The model under review builds one solid part; all positions refer to its coordinate system, in mm. A direction names the side the tool comes from. Give positions to 0.01 mm unless a question says otherwise; leave off trailing zeros. Loops run counter-clockwise (first coordinate to the right, second up) from the corner with the lowest first, then second, coordinate; pieces in that order, holes last. Notation, with made-up numbers: (-9.5, -24.5) - (8.5, -24.5) arc R25 ccw to (8.5, -10.5) - close; hole circle Ø10 at (-6.5, 74.25). An arc over 180 degrees is marked (long way). Answer as a JSON object with one key per item and string values.
from build123d import *


# Not quite as in the source:
# - a feature names something its author has since deleted; it is built from what else it names


with BuildPart() as f2:
    # F2: sweep along a path in F0
    with BuildLine(Plane.XY) as f2_path:
        Line((-7.5, -8.5), (-7.5, 8.5))
        ThreePointArc((-7.5, 8.5), (-6.0355339059, 12.0355339059), (-2.5, 13.5))
        Line((-2.5, 13.5), (2.5, 13.5))
        ThreePointArc((2.5, 13.5), (6.0355339059, 12.0355339059), (7.5, 8.5))
        Line((7.5, 8.5), (7.5, -8.5))
        ThreePointArc((7.5, -8.5), (6.0355339059, -12.0355339059), (2.5, -13.5))
        Line((2.5, -13.5), (-2.5, -13.5))
        ThreePointArc((-2.5, -13.5), (-6.0355339059, -12.0355339059), (-7.5, -8.5))
    # F1 (on Front) → F2 (sweep)
    with BuildSketch(Plane.XZ):
        Polygon((-5.751425866, 1.454347861), (-6.6942584633, 1.8659339551), (-9.2492606491, 1.454347861), (-9.3934396282, 0), (-9.2492606491, -1.454347861), (-6.6942584633, -1.8659339551), (-5.751425866, -1.454347861), (-5.751425866, 0), align=None)
    sweep(path=f2_path.line)


solid = f2.part
Q1. Consider section D-D, the plane z = -0.8. State the section outline as (x, y) points, plus the area to 3 significant figures.
Results:
{"outline": "(-9.31, -8.5) arc R6.81 ccw to (-2.5, -15.31) - (2.5, -15.31) arc R6.81 ccw to (9.31, -8.5) - (9.31, 8.5) arc R6.81 ccw to (2.5, 15.31) - (-2.5, 15.31) arc R6.81 ccw to (-9.31, 8.5) - close; hole (-5.75, -8.5) arc R3.25 ccw to (-2.5, -11.75) - (2.5, -11.75) arc R3.25 ccw to (5.75, -8.5) - (5.75, 8.5) arc R3.25 ccw to (2.5, 11.75) - (-2.5, 11.75) arc R3.25 ccw to (-5.75, 8.5) - close", "area": "269 mm^2"}
Q2. Clearance check with flat-ended pins moving along their axes: pin 1 Ø2 at (x, y) = (5.5, -7) entering from +Z; pin 2 Ø8 at (x, y) = (-5, -3.5) entering from -Z; pin 3 Ø1 at (x, z) = (6.5, 1) entering from -Y. State where each tip first meets the part, or that it passes through.
Results:
{"pin 1": "stops at z = 1.78", "pin 2": "stops at z = -1.87", "pin 3": "stops at y = -14.33"}
Q3. Consider section A-A, the plane y = 5. State the section outline as (x, z) points, plus the area to 3 significant figures.
Results:
{"outline": "(-9.39, 0) - (-9.25, -1.45) - (-6.69, -1.87) - (-5.75, -1.45) - (-5.75, 1.45) - (-6.69, 1.87) - (-9.25, 1.45) - close; (5.75, -1.45) - (6.69, -1.87) - (9.25, -1.45) - (9.39, 0) - (9.25, 1.45) - (6.69, 1.87) - (5.75, 1.45) - close", "area": "23.6 mm^2"}
Q4. For faces 1 (the face through (-4.8, 10.8, 0)), 2 (the face through (-5.94, -12.02, 1.75)), 3 (the face through (-0.035, -12.229, -1.663)), list the 3-axis set-ups (+Z, -Z, +X, -X, +Y, -Y) from which the entire face can be reached by the end or side of a thin tool; tool diameter is ignored.
Results:
{"face 1": "+Z, -Z", "face 2": "+Z, -X, -Y", "face 3": "-Z"}
Q5. To check wall thickness, follow probe 1 along X at (y, z) = (6, -0.55); probe 2 along X at (y, z) = (-9, 1.2); probe 3 along Y at (x, z) = (5.25, -0.1). State the ranges of each line that lie inside material, in increasing order. Write a range as [from, to].
Results:
{"probe 1": "x = [-9.34, -5.75], [5.75, 9.34]", "probe 2": "x = [-9.26, -5.71], [5.71, 9.26]", "probe 3": "y = [-14.81, -10.23], [10.23, 14.81]"}
Q6. The part is to be moulded in two halves that separate along Y. For faces 4 (the face through (4.8, -10.8, 0)), 5 (the face through (-0.03, -15.32, 0.74)), 6 (the face through (5.917, 11.993, -1.754)), say which applies: +Y half, -Y half, draft (parallel to the pull), parting line (faces both ways), or undercut.
Results:
{"face 4": "undercut", "face 5": "-Y half", "face 6": "+Y half"}
Q7. Consider section B-B, the plane x = 1.25. State the section outline as (y, z) points, plus the area to 3 significant figures.
Results:
{"outline": "(-15.39, 0) - (-15.25, -1.45) - (-12.69, -1.87) - (-11.75, -1.45) - (-11.75, 1.45) - (-12.69, 1.87) - (-15.25, 1.45) - close; (11.75, -1.45) - (12.69, -1.87) - (15.25, -1.45) - (15.39, 0) - (15.25, 1.45) - (12.69, 1.87) - (11.75, 1.45) - close", "area": "23.6 mm^2"}
Q8. Consider section C-C, the plane z = 0.7. State the section outline as (x, y) points.
Results:
{"outline": "(-9.32, -8.5) arc R6.82 ccw to (-2.5, -15.32) - (2.5, -15.32) arc R6.82 ccw to (9.32, -8.5) - (9.32, 8.5) arc R6.82 ccw to (2.5, 15.32) - (-2.5, 15.32) arc R6.82 ccw to (-9.32, 8.5) - close; hole (-5.75, -8.5) arc R3.25 ccw to (-2.5, -11.75) - (2.5, -11.75) arc R3.25 ccw to (5.75, -8.5) - (5.75, 8.5) arc R3.25 ccw to (2.5, 11.75) - (-2.5, 11.75) arc R3.25 ccw to (-5.75, 8.5) - close"}
